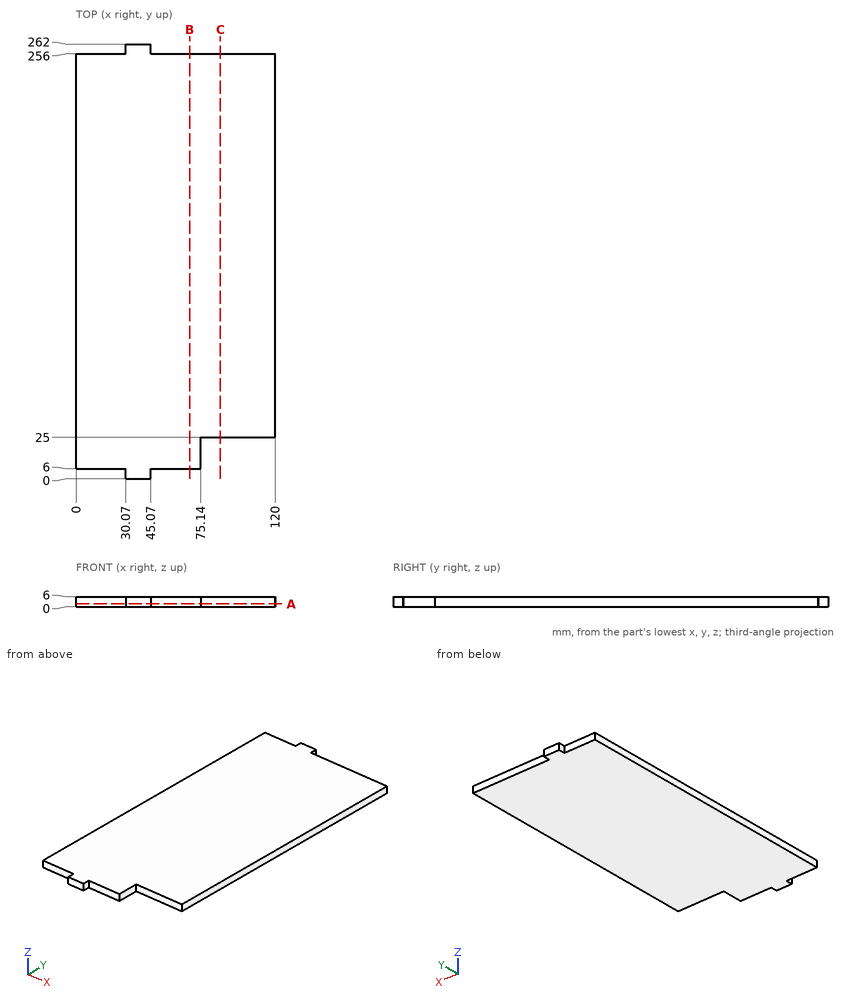
Here's the drawing with two shaded views (mm, measured from the low corner). I have some questions. Round coordinates to 2 decimals unless told otherwise and drop trailing zeros. Loops run counter-clockwise (first coordinate to the right, second up) from the corner with the lowest first, then second, coordinate; pieces in that order, holes last. Notation, with made-up numbers: M 9.5,87 L 31.5,87 A30 cw 31.5,122 Z; hole C 66,51 d8. An arc over 180 degrees is marked long. Answer as a JSON object with one key per item and string values. Group by question number.
Q1. Imagine slicing it at C-C, the plane x = 87. Please give me the cut outline in (y, z), then the cut area to 3 significant figures.
Q2. Please list where these lines run through material, in increasing order: L1, parallel to Y at x = 17, z = 3; L2, parallel to Y at x = 80.5, z = 2.05.
Q3. Will these pins go through, and if not, where does the flat tip stop? pin 1 (1.8 mm diameter, centred on y = 259, z = 2.5, fed in from -X); pin 2 (3 mm diameter, centred on x = 20.5, z = 4, fed in from +Y); pin 3 (1.8 mm diameter, centred on y = 14, z = 4, fed in from +X).
Q4. Imagine slicing it at A-A, the plane z = 1.7. Please give me the cut outline in (x, y), then the cut area to 3 significant figures.
Q5. Imagine slicing it at B-B, the plane x = 68.5. Please give me the cut outline in (y, z), then the cut area to 3 significant figures.
Findings:
{
 "1": {"outline": "M 25,0 L 256,0 L 256,6 L 25,6 Z", "area": "1,390 mm2"},
 "2": {"L1": "y = 6 to 256", "L2": "y = 25 to 256"},
 "3": {"pin 1": "stops at x = 30.07", "pin 2": "stops at y = 256", "pin 3": "stops at x = 75.14"},
 "4": {"outline": "M 0,6 L 30.07,6 L 30.07,0 L 45.07,0 L 45.07,6 L 75.14,6 L 75.14,25 L 120,25 L 120,256 L 45.07,256 L 45.07,262 L 30.07,262 L 30.07,256 L 0,256 Z", "area": "29,300 mm2"},
 "5": {"outline": "M 6,0 L 256,0 L 256,6 L 6,6 Z", "area": "1,500 mm2"}
}
